Job drawing, mm, ordinate dimensions from the low corner. One solid piece. A direction names the side the tool comes from. Give positions to 0.01 mm unless a question says otherwise; leave off trailing zeros. Write each loop counter-clockwise with the first axis right and the second up, starting at its lowest first coordinate (ties: lowest second). Pieces come first, ordered by that corner, then holes. Notation, with made-up numbers: M -27.75,61.5 L -10.75,61.5 A21 cw -10.75,82.5 Z; hole C -30,-20 d2. An arc over 180 degrees is marked long. Answer as CSV lines item,"result". Start each with the question number.
Item 1: Pin check, flat tips, straight feed: pin 1 (2.5 mm diameter, centred on x = 32.5, y = 6.75, fed in from -Z); pin 2 (1.5 mm diameter, centred on y = 3, z = 2.5, fed in from -X); pin 3 (2 mm diameter, centred on x = 6.5, y = 3, fed in from -Z); pin 4 (4 mm diameter, centred on x = 22.5, y = 10, fed in from +Z). Stop position of each tip, or through.
Item 2: Band-saw the part on B-B, the plane z = 0.75. List the corners of the cut face in (x, y).
Item 3: Wall check: L1, parallel to X at y = 6.75, z = 1.05; L2, parallel to Y at x = 31, z = 0.65; L3, parallel to X at y = 5.5, z = 1.05. Give the ranges that are in metal, low to high. Write a range as from..to.
Item 4: Band-saw the part on C-C, the plane z = 2.4. List the corners of the cut face in (x, y), then the cut area to 3 significant figures.
Item 5: Two-plate mould, pull along X, no slides. Class the marked faces 1 and 2: +X half, -X half, draft (parallel to the pull), parting line (faces both ways), or undercut.
Item 6: 3-axis set-ups, long thin cutter, end or side, ignore diameter. For the marked faces 3, 4 and 5: which of +Z, -Z, +X, -X, +Y, -Y reach the whole face in a straight line?
Item 7: Band-saw the part on A-A, the plane y = 6.75. List the corners of the cut face in (x, z), then the cut area to 3 significant figures.
Item 8: Band-saw the part on D-D, the plane y = 12.5. List the corners of the cut face in (x, z).
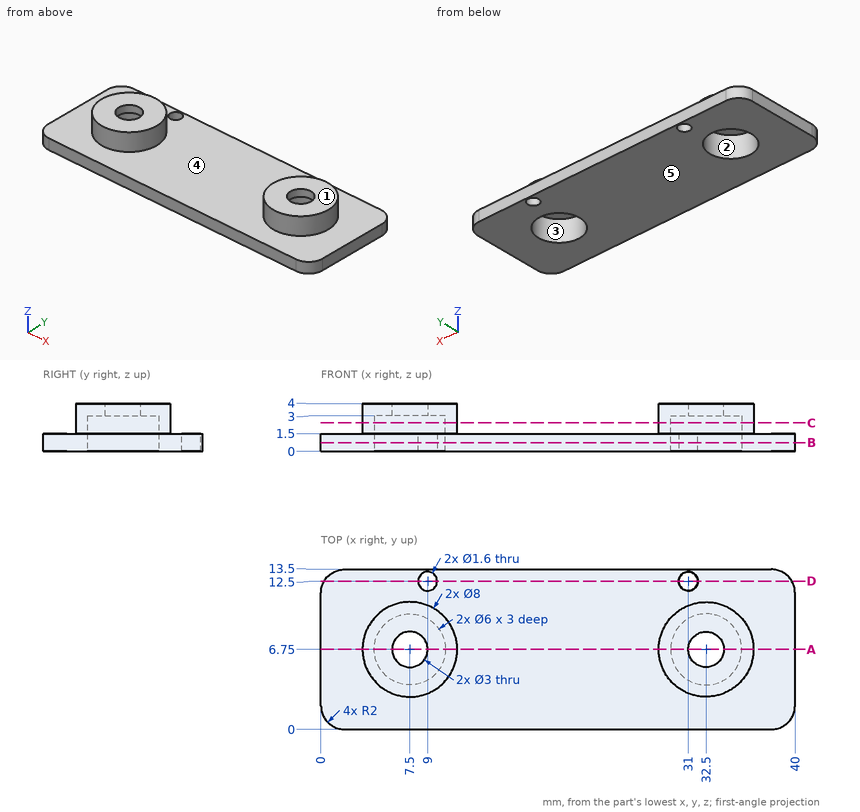
Output:
1,pin 1,"through"
1,pin 2,"x = 4.85"
1,pin 3,"z = 0"
1,pin 4,"z = 1.5"
2,outline,"M 0,2 A2 ccw 2,0 L 38,0 A2 ccw 40,2 L 40,11.5 A2 ccw 38,13.5 L 2,13.5 A2 ccw 0,11.5 Z; hole C 7.5,6.75 d6; hole C 9,12.5 d1.6; hole C 32.5,6.75 d6; hole C 31,12.5 d1.6"
3,L1,"0..4.5, 10.5..29.5, 35.5..40"
3,L2,"0..4.15, 9.35..11.7, 13.3..13.5"
3,L3,"0..4.77, 10.23..29.77, 35.23..40"
4,outline,"C 7.5,6.75 d8; C 32.5,6.75 d8; hole C 7.5,6.75 d6; hole C 32.5,6.75 d6"
4,area,"44.0 mm²"
5,face 1,"draft"
5,face 2,"undercut"
6,face 3,"-Z"
6,face 4,"+Z"
6,face 5,"-Z, +X, -X, +Y, -Y"
7,outline,"M 0,0 L 4.5,0 L 4.5,3 L 6,3 L 6,4 L 3.5,4 L 3.5,1.5 L 0,1.5 Z; M 9,3 L 10.5,3 L 10.5,0 L 29.5,0 L 29.5,3 L 31,3 L 31,4 L 28.5,4 L 28.5,1.5 L 11.5,1.5 L 11.5,4 L 9,4 Z; M 34,3 L 35.5,3 L 35.5,0 L 40,0 L 40,1.5 L 36.5,1.5 L 36.5,4 L 34,4 Z"
7,area,"58.0 mm²"
8,outline,"M 0.27,0 L 8.2,0 L 8.2,1.5 L 0.27,1.5 Z; M 9.8,0 L 30.2,0 L 30.2,1.5 L 9.8,1.5 Z; M 31.8,0 L 39.73,0 L 39.73,1.5 L 31.8,1.5 Z"
